Geometry check sheet. Reference: the model listing, model coordinates, mm. Face numbers are marked on the shaded views. Coordinates: 2 decimals unless noted, no trailing zeros. Write each loop counter-clockwise with the first axis right and the second up, starting at its lowest first coordinate (ties: lowest second). Pieces come first, ordered by that corner, then holes.
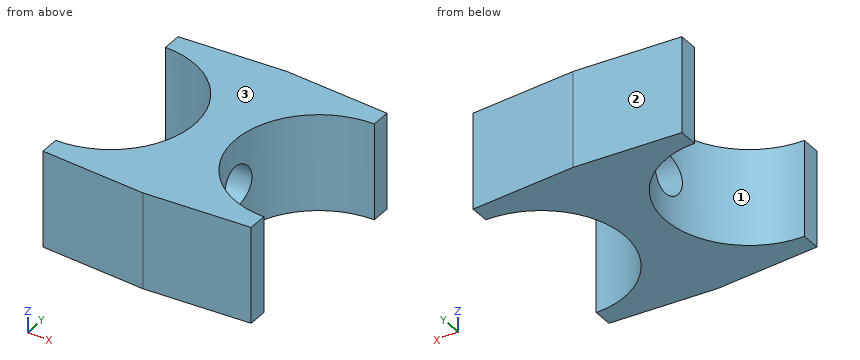
from build123d import *

# Parameters (mm, degrees)
F1_DEPTH = 7.5
F2_DEPTH = 12.5
F3_DEPTH = 12.5
F4_R     = 3.3
F4_R_2   = 3.05
F5_DEPTH = 25


with BuildPart() as f1:
    # F0 (on Top) → F1 (new body, symmetric)
    with BuildSketch(Plane.XY):
        with BuildLine():
            ThreePointArc((16.2, -16), (0.200029, 0.030397), (16.260794, 15.999885))
            Line((16.260794, 15.999885), (0, 17))
            Line((0, 17), (0, -17))
            Line((0, -17), (16.2, -16))
        make_face()
        with BuildLine():
            Line((16.255094, 12.999883), (16.260794, 15.999885))
            ThreePointArc((16.260794, 15.999885), (0.200029, 0.030397), (16.2, -16))
            Line((16.2, -16), (16.205699, -12.999999))
            ThreePointArc((16.205699, -12.999999), (3.200023, 0.024697), (16.255094, 12.999883))
        make_face()
        with BuildLine():
            Line((16.205699, -12.999999), (16.255094, 12.999883))
            ThreePointArc((16.255094, 12.999883), (3.200023, 0.024697), (16.205699, -12.999999))
        make_face()
        with BuildLine():
            Line((0, -17), (0, 17))
            Line((0, 17), (-16.260794, 15.999885))
            ThreePointArc((-16.260794, 15.999885), (-0.200029, 0.030397), (-16.2, -16))
            Line((-16.2, -16), (0, -17))
        make_face()
        with BuildLine():
            ThreePointArc((-16.2, -16), (-0.200029, 0.030397), (-16.260794, 15.999885))
            Line((-16.260794, 15.999885), (-16.255094, 12.999883))
            ThreePointArc((-16.255094, 12.999883), (-3.200023, 0.024697), (-16.205699, -12.999999))
            Line((-16.205699, -12.999999), (-16.2, -16))
        make_face()
        with BuildLine():
            ThreePointArc((-16.205699, -12.999999), (-3.200023, 0.024697), (-16.255094, 12.999883))
            Line((-16.255094, 12.999883), (-16.205699, -12.999999))
        make_face()
    extrude(amount=F1_DEPTH, both=True)

    # F0 (on Top) → F2 (cut, symmetric)
    with BuildSketch(Plane.XY):
        with BuildLine():
            ThreePointArc((-16.205699, -12.999999), (-3.200023, 0.024697), (-16.255094, 12.999883))
            Line((-16.255094, 12.999883), (-16.205699, -12.999999))
        make_face()
    extrude(amount=F2_DEPTH, both=True, mode=Mode.SUBTRACT)

    # F0 (on Top) → F3 (cut, symmetric)
    with BuildSketch(Plane.XY):
        with BuildLine():
            Line((16.205699, -12.999999), (16.255094, 12.999883))
            ThreePointArc((16.255094, 12.999883), (3.200023, 0.024697), (16.205699, -12.999999))
        make_face()
    extrude(amount=F3_DEPTH, both=True, mode=Mode.SUBTRACT)

    # F4 (on face) → F5 (cut)
    with BuildSketch(Plane(origin=(16.230338, -0.030835, 0), x_dir=(0.0019, 0.999998, 0), z_dir=(0.999998, -0.0019, 0))):
        Circle(F4_R)
        Circle(F4_R_2, mode=Mode.SUBTRACT)
        Circle(F4_R_2)
    extrude(amount=-F5_DEPTH, mode=Mode.SUBTRACT)


solid = f1.part
1. Thickness scan on line 1 along Y through (x, z) = (8.5, -2.25); line 2 along Z through (x, y) = (2.5, 3); line 3 along Y through (x, z) = (11.5, -6.5). Record the ranges inside material, lowest first.
Computed values:
line 1: y = -16.48 to -10.47, 10.47 to 16.48
line 2: z = -7.5 to -1.36, 1.36 to 7.5
line 3: y = -16.29 to -12.12, 12.12 to 16.29
2. Sectioned sample at D-D, the plane z = -1.75. Record the boundary of the cut face in (x, y).
Computed values:
outline: (-16.26, 13) arc R13 cw to (-3.51, 2.8) - (3.5, 2.79) arc R13 cw to (16.26, 13) - (16.26, 16) - (0, 17) - (-16.26, 16) - close; (-16.21, -13) - (-16.2, -16) - (0, -17) - (16.2, -16) - (16.21, -13) arc R13 cw to (3.51, -2.8) - (-3.5, -2.79) arc R13 cw to start
3. Sectioned sample at C-C, the plane x = -11.5. Record the boundary of the cut face in (y, z), and give its area (3 significant figures).
Computed values:
outline: (-16.29, -7.5) - (-12.12, -7.5) - (-12.12, 7.5) - (-16.29, 7.5) - close; (12.12, -7.5) - (16.29, -7.5) - (16.29, 7.5) - (12.12, 7.5) - close
area: 125 mm2
4. Sectioned sample at B-B, the plane z = 2.5. Record the boundary of the cut face in (x, y), and give its area (3 significant figures).
Computed values:
outline: (-16.26, 13) arc R13 cw to (-3.38, 2.16) - (3.38, 2.15) arc R13 cw to (16.26, 13) - (16.26, 16) - (0, 17) - (-16.26, 16) - close; (-16.21, -13) - (-16.2, -16) - (0, -17) - (16.2, -16) - (16.21, -13) arc R13 cw to (3.38, -2.16) - (-3.38, -2.15) arc R13 cw to start
area: 511 mm2
5. Draft check along Y on the marked faces 1, 2 and 3. Enter one of: released by +Y, released by -Y, zero draft, split by the parting line, or undercut.
Computed values:
face 1: undercut
face 2: released by +Y
face 3: zero draft
6. Sectioned sample at A-A, the plane x = 9.5. Record the boundary of the cut face in (y, z).
Computed values:
outline: (-16.41, -7.5) - (-11.14, -7.5) - (-11.14, 7.5) - (-16.41, 7.5) - close; (11.14, -7.5) - (16.42, -7.5) - (16.42, 7.5) - (11.14, 7.5) - close
7. Gauge pin test, flat ends, axial feed: pin 1 Ø5 at (x, z) = (10.5, -2) entering from -Y; pin 2 Ø2 at (x, z) = (10.5, -4) entering from +Y; pin 3 Ø6 at (x, z) = (-8.5, -2.5) entering from +Y. Record the tip position at first contact, or that the pin passes through.
Computed values:
pin 1: stops at y = -16.51
pin 2: stops at y = 16.42
pin 3: stops at y = 16.66
